CAD build for the part. Positions are in the model's coordinates, mm. A direction names the side the tool comes from. Give positions to 0.01 mm unless a question says otherwise; leave off trailing zeros. Write each loop counter-clockwise with the first axis right and the second up, starting at its lowest first coordinate (ties: lowest second). Pieces come first, ordered by that corner, then holes. Notation, with made-up numbers: (85, 45) - (103, 45) arc R33 cw to (103, 74) - close; hole circle Ø6 at (-24.5, 34). An arc over 180 degrees is marked (long way). Put each result on its own line as item: value. Start each with the question number.
1. Cut at B-B on z = -5. List the corners of the cut face in (x, y).
2. Cut at D-D on z = -7.75. List the corners of the cut face in (x, y).
3. Drop flat-ended pins along their axis: pin 1 (5 mm diameter, centred on y = 10, z = -7, fed in from +X) (3 decimals); pin 2 (1.5 mm diameter, centred on x = -0.5, z = 5, fed in from +Y); pin 3 (1 mm diameter, centred on x = -5.5, y = 4, fed in from -Z); pin 4 (1.5 mm diameter, centred on x = -3, y = 4.5, fed in from -Z). Give the stop position or say it passes through.
4. Cut at C-C on y = 5. List the corners of the cut face in (x, z) (3 decimals).
5. Mould opens along X. For faces 3 (the flat face through (6.4, 12.7, -2.8)), 4 (the flat face through (5.856, 6.261, 3.318)), 5 (the cylindrical face through (7.559, 6.261, 5.796)) say: +X half, -X half, draft (parallel to the pull), parting line (faces both ways), or undercut.
6. Wall check: line 1 (Z direction, x = 1.5, y = 10.75); line 2 (X direction, y = 6.25, z = 0.75); line 3 (X direction, y = 9.5, z = 4.75). Give the ranges that are in metal, low to high.
7. Cut at A-A on x = 0. List the corners of the cut face in (y, z) (3 decimals), and give its area (3 significant figures).
8. Tool access for faces 1 (the flat face through (6.4, 0, -2.8)), 2 (the flat face through (0, 6, 6.731)): list every direction of +Z, -Z, +X, -X, +Y, -Y with a clear straight run to the whole face (end or side of a thin tool).
Autodesk Inventor part; units mm, degrees
ref_plane "YZ Plane" through (0, 0, 0) normal (1, 0, 0) x (0, 1, 0)
ref_plane "XZ Plane" through (0, 0, 0) normal (0, 1, 0) x (-1, 0, 0)
ref_plane "XY Plane" through (0, 0, 0) normal (0, 0, 1) x (1, 0, 0)
sketch "Sketch1" plane through (0, 0, 0) normal (0, 1, 0) x (-1, 0, 0)
  line L0 (-3.8861, 6.731) -> (3.8861, 6.731)
  line L1 (3.8861, 6.731) -> (7.7723, 0)
  line L2 (7.7723, 0) -> (3.8861, -6.731)
  line L3 (3.8861, -6.731) -> (-3.8861, -6.731)
  line L4 (-3.8861, -6.731) -> (-7.7723, 0)
  line L5 (-7.7723, 0) -> (-3.8861, 6.731)
  circle A0 centre (0, 0) radius 9.525
  point P0 (5.8292, -3.3655)
  dimension "d0" = 13.462
  dimension "d1" = 19.05
extrude "Extrusion1" add sketch "Sketch1" along normal blind 12.7
properties part number "SP-003"
Report:
1. outline: (-8.11, 0) - (-4.89, 0) - (-4.89, 12.7) - (-8.11, 12.7) - close; (4.89, 0) - (8.11, 0) - (8.11, 12.7) - (4.89, 12.7) - close
2. outline: (-5.54, 0) - (5.54, 0) - (5.54, 12.7) - (-5.54, 12.7) - close
3. pin 1: stops at x = 8.395
3. pin 2: passes through
3. pin 3: stops at z = -8.11
3. pin 4: stops at z = -9.26
4. outline: circle Ø19.05 at (0, 0); hole (-7.772, 0) - (-3.886, -6.731) - (3.886, -6.731) - (7.772, 0) - (3.886, 6.731) - (-3.886, 6.731) - close
5. face 3: draft
5. face 4: undercut
5. face 5: parting line
6. line 1: z = -9.41 to -6.73, 6.73 to 9.41
6. line 2: x = -9.5 to -7.34, 7.34 to 9.5
6. line 3: x = -8.26 to -5.03, 5.03 to 8.26
7. outline: (0, -9.525) - (12.7, -9.525) - (12.7, -6.731) - (0, -6.731) - close; (0, 6.731) - (12.7, 6.731) - (12.7, 9.525) - (0, 9.525) - close
7. area: 71.0 mm²
8. face 1: +Z, -Z, +X, -X, -Y
8. face 2: +Y, -Y
